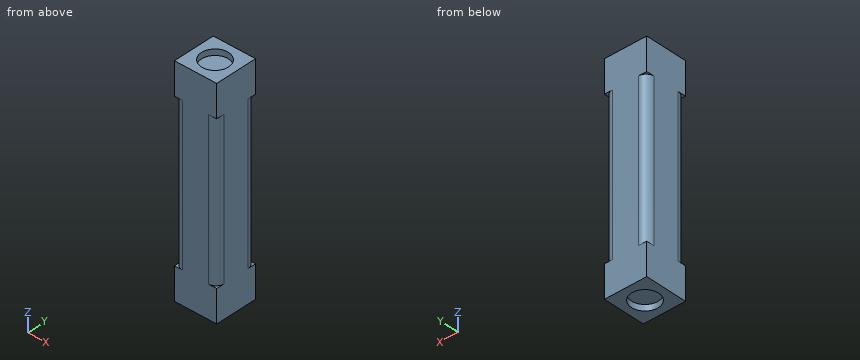
```python
from build123d import *

# Parameters (mm, degrees)
SKETCH_W        = 15.75
SKETCH_H        = 15.75
PAD_DEPTH       = 12
PAD001_DEPTH    = 57.35
SKETCH002_W     = 15.75
SKETCH002_H     = 15.75
PAD002_DEPTH    = 12
SKETCH003_R     = 5.05
POCKET_DEPTH    = 2.2
SKETCH004_R     = 5.05
POCKET001_DEPTH = 2.2


with BuildPart() as part:
    # Sketch → Pad (new body)
    with BuildSketch(Plane.XY):
        Rectangle(SKETCH_W, SKETCH_H)
    extrude(amount=PAD_DEPTH)

    # Sketch001 → Pad001 (join)
    with BuildSketch(Plane.XY.offset(12)):
        with BuildLine():
            Line((-4.875, -7.875), (4.875, -7.875))
            ThreePointArc((4.875, -7.875), (6.99632, -6.99632), (7.875, -4.875))
            Line((7.875, -4.875), (7.875, 4.875))
            ThreePointArc((7.875, 4.875), (6.99632, 6.99632), (4.875, 7.875))
            Line((4.875, 7.875), (-4.875, 7.875))
            ThreePointArc((-4.875, 7.875), (-6.99632, 6.99632), (-7.875, 4.875))
            Line((-7.875, 4.875), (-7.875, -4.875))
            ThreePointArc((-7.875, -4.875), (-6.99632, -6.99632), (-4.875, -7.875))
        make_face()
    extrude(amount=PAD001_DEPTH)

    # Sketch002 (on Face15 of Pad001) → Pad002 (join)
    with BuildSketch(Plane.XY.offset(69.35)):
        Rectangle(SKETCH002_W, SKETCH002_H)
    extrude(amount=PAD002_DEPTH)

    # Sketch003 (on Face7 of Pad002) → Pocket (cut)
    with BuildSketch(Plane.XY.offset(81.35)):
        Circle(SKETCH003_R)
    extrude(amount=-POCKET_DEPTH, mode=Mode.SUBTRACT)

    # Sketch004 → Pocket001 (cut)
    with BuildSketch(Plane.XY):
        Circle(SKETCH004_R)
    extrude(amount=POCKET001_DEPTH, mode=Mode.SUBTRACT)


solid = part.part
```
Check sheet for the modelled part. Datum: model origin and axes. Units: mm. Round coordinates to 2 decimals unless told otherwise and drop trailing zeros. Order: outer loops, then holes, each group sorted by start corner. A loop starts at its lowest first (then second) coordinate and runs counter-clockwise, first axis right, second up. Notation, with made-up numbers: (46, -7) -> (88, -7) arc R16 ccw to (88, 14) -> close; hole circle Ø1 at (-1.5, 60.5). An arc over 180 degrees is marked (long way). One line per item, written item: value. Start each with the question number.
Q1. Cross-section at B-B (z = 66). Record the boundary of the cut face in (x, y) (3 decimals).
Q2. Thickness scan on line 1 (Y direction, x = 0, z = 1.6) (3 decimals); line 2 (Z direction, x = 2.5, y = 1.25); line 3 (X direction, y = 5.5, z = 33.5). Record the ranges inside material, lowest first.
Q3. Cross-section at A-A (y = 0). Record the boundary of the cut face in (x, z) (3 decimals), and give its area (3 significant figures).
Q4. Gauge pin test, flat end, axial feed: pin 1 Ø8 at (x, y) = (0, -0.5) entering from +Z. Record the tip position at first contact, or that the pin passes through.
Completed:
1. outline: (-7.875, -4.875) arc R3 ccw to (-4.875, -7.875) -> (4.875, -7.875) arc R3 ccw to (7.875, -4.875) -> (7.875, 4.875) arc R3 ccw to (4.875, 7.875) -> (-4.875, 7.875) arc R3 ccw to (-7.875, 4.875) -> close
2. line 1: y = -7.875 to -5.05, 5.05 to 7.875
2. line 2: z = 2.2 to 79.15
2. line 3: x = -7.81 to 7.81
3. outline: (-7.875, 0) -> (-5.05, 0) -> (-5.05, 2.2) -> (5.05, 2.2) -> (5.05, 0) -> (7.875, 0) -> (7.875, 81.35) -> (5.05, 81.35) -> (5.05, 79.15) -> (-5.05, 79.15) -> (-5.05, 81.35) -> (-7.875, 81.35) -> close
3. area: 1,240 mm²
4. pin 1: stops at z = 79.15
